Verification items for the finished model (mm, model axes). Face numbers are marked on the shaded views. A direction names the side the tool comes from. Round coordinates to 2 decimals unless told otherwise and drop trailing zeros. Order: outer loops, then holes, each group sorted by start corner. A loop starts at its lowest first (then second) coordinate and runs counter-clockwise, first axis right, second up. Notation, with made-up numbers: M 57.5,45.25 L 71.5,45.25 A17 cw 71.5,55.25 Z; hole C -32,73.25 d1. An arc over 180 degrees is marked long. Return JSON: item names as keys, results as strings. Group by question number.
from build123d import *

# Parameters (mm, degrees)
F0_R      = 8.382
F1_DEPTH  = 6.731
F2_W      = 114.3
F2_H      = 177.8
F3_DEPTH  = 11.3284
F4_R      = 21.971
F5_DEPTH  = 15.875
F6_W      = 66.04
F6_H      = 10.16
F7_DEPTH  = 177.8
F8_SIZE   = 60.96
F10_DEPTH = 95.632


# Not quite as in the source:
# - a pattern or mirror of a feature is missing from the dataset's text; its kind, count and spacing are read off the source's solid


with BuildPart() as f1:
    # F0 (on Top) → F1 (new body, symmetric)
    with BuildSketch(Plane.XY):
        with BuildLine():
            Line((177.8, 139.7), (-177.8, 139.7))
            ThreePointArc((-177.8, 139.7), (-195.7605122421, 132.2605122421), (-203.2, 114.3))
            Line((-203.2, 114.3), (-203.2, -114.3))
            ThreePointArc((-203.2, -114.3), (-195.7605122421, -132.2605122421), (-177.8, -139.7))
            Line((-177.8, -139.7), (177.8, -139.7))
            ThreePointArc((177.8, -139.7), (195.7605122421, -132.2605122421), (203.2, -114.3))
            Line((203.2, -114.3), (203.2, 114.3))
            ThreePointArc((203.2, 114.3), (195.7605122421, 132.2605122421), (177.8, 139.7))
        make_face()
        with Locations((-82.55, -82.55)):
            Circle(F0_R, mode=Mode.SUBTRACT)
        with Locations((82.55, -82.55)):
            Circle(F0_R, mode=Mode.SUBTRACT)
        with Locations((-82.55, 82.55)):
            Circle(F0_R, mode=Mode.SUBTRACT)
        with Locations((82.55, 82.55)):
            Circle(F0_R, mode=Mode.SUBTRACT)
    extrude(amount=F1_DEPTH, both=True)

    # F2 (on face) → F3 (join)
    with BuildSketch(Plane(origin=(-203.2, 0, 0), x_dir=(0, -1, 0), z_dir=(-1, 0, 0))):
        Rectangle(F2_W, F2_H)
    f3 = extrude(amount=-F3_DEPTH)

    # F3_copies: F3 across plane
    add(f3.mirror(Plane(origin=(0, 0, 0), x_dir=(0, 0, 1), z_dir=(1, 0, 0))))

    # F4 (on Front) → F5 (join, symmetric)
    with BuildSketch(Plane.XZ):
        with BuildLine():
            ThreePointArc((-223.52, 88.9), (-244.6799408534, 57.8520750061), (-273.9982965787, 34.354186571))
            ThreePointArc((-273.9982965787, 34.354186571), (-293.751, 0), (-273.9982965787, -34.354186571))
            ThreePointArc((-273.9982965787, -34.354186571), (-244.6799408534, -57.8520750061), (-223.52, -88.9))
            Line((-223.52, -88.9), (-203.2, -88.9))
            Line((-203.2, -88.9), (-203.2, -6.731))
            Line((-203.2, -6.731), (-203.2, 6.731))
            Line((-203.2, 6.731), (-203.2, 88.9))
            Line((-203.2, 88.9), (-223.52, 88.9))
        make_face()
        with Locations((-254, 0)):
            Circle(F4_R, mode=Mode.SUBTRACT)
    f5 = extrude(amount=F5_DEPTH, both=True)

    # F5_copies: F5 across plane
    add(f5.mirror(Plane(origin=(0, 0, 0), x_dir=(0, 0, 1), z_dir=(1, 0, 0))))

    # F6 (on face) → F7 (join, through all)
    with BuildSketch(Plane.XY.offset(88.9)):
        with Locations((-158.8516, 0)):
            Rectangle(F6_W, F6_H)
    f7 = extrude(amount=-F7_DEPTH)

    # F7_copies: F7 across plane
    add(f7.mirror(Plane(origin=(0, 0, 0), x_dir=(0, 0, 1), z_dir=(1, 0, 0))))

    # F8
    f8_edges = [f1.edges().sort_by_distance(p)[0] for p in [
        (-125.8316, 0, -88.9),
        (-125.8316, 0, 88.9),
        (125.8316, 0, -88.9),
        (125.8316, 0, 88.9),
    ]]
    chamfer(f8_edges, length=F8_SIZE)

    # F9 (on face) → F10 (cut, through all)
    with BuildSketch(Plane(origin=(0, 0, -6.731), x_dir=(1, 0, 0), z_dir=(0, 0, -1))):
        with BuildLine():
            Line((-95.25, -29.5275), (-59.6566653523, -47.4080402362))
            ThreePointArc((-59.6566653523, -47.4080402362), (-2.9560938308, -76.1426392323), (55.8015879509, -51.8904883592))
            Line((55.8015879509, -51.8904883592), (95.25, -29.5275))
            Line((95.25, -29.5275), (95.25, 29.5275))
            Line((95.25, 29.5275), (61.3953822556, 45.1336574818))
            ThreePointArc((61.3953822556, 45.1336574818), (-1.0966393905, 76.1921083974), (-62.6689060075, 43.3479898015))
            Line((-62.6689060075, 43.3479898015), (-95.25, 29.5275))
            Line((-95.25, 29.5275), (-95.25, -29.5275))
        make_face()
    extrude(amount=-F10_DEPTH, mode=Mode.SUBTRACT)


solid = f1.part
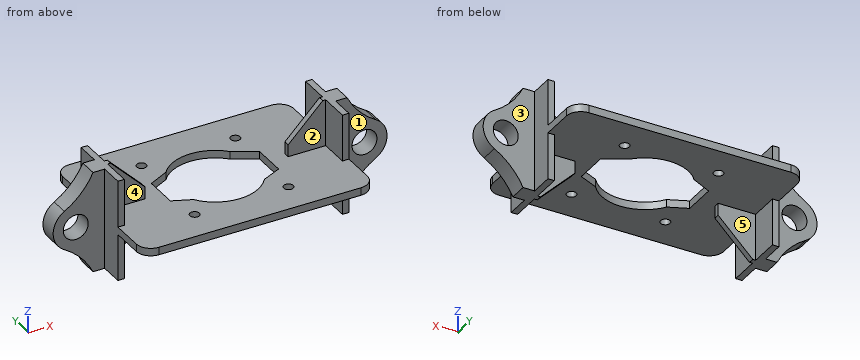
1. Cross-section at B-B (x = 82.55). Enter the section's corners in (y, z), plus the area to 3 significant figures.
2. Thickness scan on line 1 along X through (y, z) = (82, 2); line 2 along X through (y, z) = (36, -61); line 3 along Y through (x, z) = (-82.55, -4). Record the ranges inside material, lowest first. Write a range as from..to.
3. Cross-section at C-C (z = -54). Enter the section's corners in (x, y) (3 decimals), plus the area to 3 significant figures.
4. Draft check along X on the marked faces 1 and 2. Enter one of: +X half, -X half, draft (parallel to the pull), parting line (faces both ways), or undercut.
5. Access from +Z, -Z, +X, -X, +Y, -Y to the whole of each face (thin tool, end or side, straight path). Record for the marked faces 3, 4 and 5.
6. Go/stop test with flat-tipped pins: pin 1 (3.5 mm diameter, centred on x = 196, z = 29, fed in from +Y); pin 2 (5 mm diameter, centred on y = 9.5, z = -19, fed in from +X); pin 3 (3 mm diameter, centred on y = 2.5, z = -14, fed in from -X). Record where each tip stops, or that it passes through.
7. Cross-section at D-D (x = -166.5). Enter the section's corners in (y, z), plus the area to 3 significant figures.
8. Cross-section at A-A (y = 82.55). Enter the section's corners in (x, z), plus the area to 3 significant figures.
Computed:
{
 "1": {"outline": "M -139.7,-6.73 L -90.93,-6.73 L -90.93,6.73 L -139.7,6.73 Z; M -74.17,-6.73 L -35.38,-6.73 L -35.38,6.73 L -74.17,6.73 Z; M 36.73,-6.73 L 74.17,-6.73 L 74.17,6.73 L 36.73,6.73 Z; M 90.93,-6.73 L 139.7,-6.73 L 139.7,6.73 L 90.93,6.73 Z", "area": "2,340 mm²"},
 "2": {"line 1": "x = -203.2..-90.91, -74.19..74.19, 90.91..203.2", "line 2": "x = -203.2..-191.87, 191.87..203.2", "line 3": "y = -139.7..-90.93, -74.17..-34.91, 35.91..74.17, 90.93..139.7"},
 "3": {"outline": "M -248.399,-15.875 L -203.2,-15.875 L -203.2,-57.15 L -191.872,-57.15 L -191.872,-5.08 L -151.892,-5.08 L -151.892,5.08 L -191.872,5.08 L -191.872,57.15 L -203.2,57.15 L -203.2,15.875 L -248.399,15.875 Z; M 151.892,-5.08 L 191.872,-5.08 L 191.872,-57.15 L 203.2,-57.15 L 203.2,-15.875 L 248.399,-15.875 L 248.399,15.875 L 203.2,15.875 L 203.2,57.15 L 191.872,57.15 L 191.872,5.08 L 151.892,5.08 Z", "area": "6,270 mm²"},
 "4": {"face 1": "draft", "face 2": "undercut"},
 "5": {"face 3": "+Z, -Z, +X, +Y", "face 4": "+Z, -Y", "face 5": "-Z, +Y"},
 "6": {"pin 1": "stops at y = 57.15", "pin 2": "stops at x = 290.16", "pin 3": "stops at x = -291.73"},
 "7": {"outline": "M -139.7,-6.73 L -5.08,-6.73 L -5.08,-68.61 L 5.08,-68.61 L 5.08,-6.73 L 139.7,-6.73 L 139.7,6.73 L 5.08,6.73 L 5.08,68.61 L -5.08,68.61 L -5.08,6.73 L -139.7,6.73 Z", "area": "5,020 mm²"},
 "8": {"outline": "M -203.2,-6.73 L -90.93,-6.73 L -90.93,6.73 L -203.2,6.73 Z; M -74.17,-6.73 L 74.17,-6.73 L 74.17,6.73 L -74.17,6.73 Z; M 90.93,-6.73 L 203.2,-6.73 L 203.2,6.73 L 90.93,6.73 Z", "area": "5,020 mm²"}
}
